The listing builds one solid part. Answer for the finished solid, in the listing's coordinates (mm). A direction names the side the tool comes from. Give positions to 0.01 mm unless a question says otherwise; leave off trailing zeros. Write each loop counter-clockwise with the first axis right and the second up, starting at its lowest first coordinate (ties: lowest second). Pieces come first, ordered by that corner, then holes. Notation, with made-up numbers: (-37.75, -26.5) - (-31.75, -26.5) arc R29 ccw to (-31.75, 5.5) - close; hole circle Ø7 at (40.25, 85.25). An arc over 180 degrees is marked (long way). One line per item, written item: value. Start each with the question number.
Autodesk Inventor part; units mm, degrees
ref_plane "XZ Plane" through (0, 0, 0) normal (0, 1, 0) x (-1, 0, 0)
ref_plane "XY Plane" through (0, 0, 0) normal (0, 0, 1) x (1, 0, 0)
sketch "Sketch1" plane through (0, 0, 0) normal (0, 0, 1) x (1, 0, 0)
  line L0 (0, 0) -> (-273.05, 0)
  line L1 (-273.05, 0) -> (-273.05, 101.6)
  line L2 (-273.05, 101.6) -> (-269.875, 101.6)
  line L3 (-269.875, 101.6) -> (-269.875, 3.175)
  line L4 (0, 0) -> (0, 3.175) construction
  line L5 (0, 3.175) -> (-269.875, 3.175)
  line L6 (0, 0) -> (273.05, 0)
  line L7 (273.05, 0) -> (273.05, 101.6)
  line L8 (273.05, 101.6) -> (269.875, 101.6)
  line L9 (269.875, 101.6) -> (269.875, 3.175)
  line L10 (0, 3.175) -> (269.875, 3.175)
  dimension "d0" = 101.6
  dimension "d1" = 273.05
  dimension "d2" = 3.175
  dimension "d4" = 3.175
extrude "Extrusion1" add sketch "Sketch1" along normal mid plane 520.7
fillet "Fillet1" radius 0.7937 2 edges at (-269.875, 3.175, 0) (269.875, 3.175, 0)
sketch "Sketch5" plane through (-269.875, 101.6, 260.35) normal (1, 0, 0) x (0, 0, -1)
  circle A0 centre (12.7, -30.1625) radius 2.5527
  circle A1 centre (22.225, -20.6375) radius 2.5527
  circle A2 centre (31.75, -11.1125) radius 2.5527
  circle A3 centre (50.8, -11.1125) radius 3.3782
  circle A4 centre (76.2, -11.1125) radius 3.7287
  circle A5 centre (12.7, -84.1375) radius 2.667
  circle A6 centre (22.225, -74.6125) radius 2.667
  circle A7 centre (31.75, -65.0875) radius 2.5527
  circle A8 centre (50.8, -77.7875) radius 3.8163
  circle A9 centre (76.2, -84.1375) radius 3.3782
  circle A10 centre (101.4806, -88.9127) radius 3.3782
  circle A11 centre (212.631, -88.9127) radius 3.3782
  circle A12 centre (228.6, -84.1375) radius 3.7287
  circle A13 centre (279.4, -81.5975) radius 3.8163
  circle A14 centre (228.6, -11.1125) radius 3.3782
  circle A15 centre (254, -11.1125) radius 3.7287
  circle A16 centre (279.4, -11.1125) radius 3.3782
  circle A17 centre (304.8, -11.1125) radius 3.3782
  circle A18 centre (330.2, -11.1125) radius 3.7287
  circle A19 centre (355.6, -11.1125) radius 3.3782
  circle A20 centre (381, -11.1125) radius 3.3782
  circle A21 centre (431.8, -11.1125) radius 3.7287
  circle A22 centre (454.025, -14.2875) radius 3.8163
  circle A23 centre (508, -77.7875) radius 3.8163
  circle A24 centre (457.2, -84.1375) radius 3.3782
  circle A25 centre (431.8, -84.1375) radius 3.7287
  circle A26 centre (475.0995, -39.081) radius 3.3782
  circle A27 centre (412.75, -38.1) radius 2.5527
  circle A28 centre (403.225, -47.625) radius 2.667
  circle A29 centre (393.7, -57.15) radius 2.5527
  circle A30 centre (381, -84.1375) radius 3.3782
  circle A31 centre (355.6, -84.1375) radius 3.3782
  circle A32 centre (330.2, -84.1375) radius 3.7287
  circle A33 centre (304.8, -84.1375) radius 3.3782
  circle A34 centre (492.125, -77.7875) radius 4.826
  circle A35 centre (508, -77.7875) radius 5.2255
  point P0 (260.35, -101.6)
extrude "Extrusion2" cut sketch "Sketch5" against normal through all contours A0 | A1 | A2 | A3 | A4 | A5 | A6 | A7 | A8 | A9 | A10 | A11 | A12 | A13 | A14 | A15 | A16 | A17 | A18 | A19 | A20 | A21 | A22 | A23 | A24 | A25 | A26 | A27 | A28 | A29 | A30 | A31 | A32 | A33 | A34
sketch "Sketch6" plane through (-269.875, 101.6, 260.35) normal (1, 0, 0) x (0, 0, -1)
  line L0 (0, 0) -> (520.7, 0)
  line L1 (0, -101.6) -> (520.7, -101.6)
  line L2 (82.55, 0) -> (234.95, 0)
  line L3 (234.95, 0) -> (234.95, -101.6)
  line L4 (234.95, -101.6) -> (82.55, -101.6)
  line L5 (82.55, -101.6) -> (82.55, 0)
  line L6 (0, 0) -> (0, -101.6)
  point P0 (260.35, -101.6)
  dimension "d18" = 82.55
  dimension "d19" = 234.95
extrude "Extrusion3" cut sketch "Sketch6" against normal through all contours L0 L3 L1 L5
properties part number "SheetBottomFloorV01saved01" material "Aluminum 6061"
Item 1: For faces 1 (the flat face through (-269.875, 53, 218)), 2 (the flat face through (-273.05, 50, 218)), determine the directions among +Z, -Z, +X, -X, +Y, -Y from which every point of the face is accessible in a straight line to the end or side of a thin tool.
Item 2: Straight lines are drawn through the part: line 1 along Y through (x, z) = (-270.95, -95.25); line 2 along Y through (x, z) = (-271.25, -171.45); line 3 along X through (y, z) = (20.5, 19.5) (3 decimals). For each, find the intervals that lie inside material, in ascending order.
Item 3: Find section A-A on z = 115.5. Determine the outline of the cut face in (x, y) (3 decimals).
Item 4: Each of these flat-tipped pins is pushed along its axis until it touches: pin 1 Ø1 at (y, z) = (26, 78.5) entering from -X (3 decimals); pin 2 Ø6 at (y, z) = (80.96, 238.12) entering from -X; pin 3 Ø1.2 at (y, z) = (1.5, 116) entering from -X (3 decimals); pin 4 Ø4 at (x, z) = (-116.5, 194) entering from +Y (3 decimals). Where does it stop, or does it pass through?
Item 5: Find section B-B on x = 81. Determine the outline of the cut face in (y, z) (3 decimals), plus the area to 3 significant figures.
Item 6: The mould has two halves that part along X. Classify faces 3 (the flat face through (-269.875, 53, -119)), 4 (the flat face through (273.05, 50, -4)), 5 (the flat face through (4, 0, -4)): +X half, -X half, draft (parallel to the pull), parting line (faces both ways), or undercut.
Values:
1. face 1: +Z, -Z, +Y
1. face 2: +Z, -Z, -X, +Y, -Y
2. line 1: 0 to 14.08, 20.84 to 87.11, 93.87 to 101.6
2. line 2: 0 to 13.73, 21.19 to 86.76, 94.22 to 101.6
2. line 3: -273.05 to -269.875, 269.875 to 273.05
3. outline: (-269.875, 0) - (273.05, 0) - (273.05, 101.6) - (269.875, 101.6) - (269.875, 3.969) arc R0.794 cw to (269.081, 3.175) - (-269.081, 3.175) arc R0.794 cw to (-269.875, 3.969) - close
4. pin 1: x = 269.875
4. pin 2: x = -273.05
4. pin 3: x = -269.875
4. pin 4: y = 3.175
5. outline: (0, -260.35) - (3.175, -260.35) - (3.175, 260.35) - (0, 260.35) - close
5. area: 1,650 mm^2
6. face 3: undercut
6. face 4: +X half
6. face 5: draft
